Build history of the part. All positions in model axes, mm. A direction names the side the tool comes from. Give positions to 0.01 mm unless a question says otherwise; leave off trailing zeros. Order: outer loops, then holes, each group sorted by start corner. A loop starts at its lowest first (then second) coordinate and runs counter-clockwise, first axis right, second up. Notation, with made-up numbers: M -12.75,-36.5 L 13.25,-36.5 A20 ccw 13.25,-13.5 Z; hole C 58.25,-27.5 d8. An arc over 180 degrees is marked long. One line per item, written item: value.
from build123d import *

# Parameters (mm, degrees)
F1_DEPTH = 8.89


with BuildPart() as f1:
    # F0 (on Top) → F1 (new body)
    with BuildSketch(Plane.XY):
        with BuildLine():
            ThreePointArc((-31.581117, 0.265729), (-27.699647, 0.639888), (-23.961117, 1.748585))
            Line((-23.961117, 1.748585), (-23.961117, -30.38213))
            ThreePointArc((-23.961117, -30.38213), (-6.162074, -48.181174), (11.636969, -30.38213))
            Line((11.636969, -30.38213), (11.636969, -17.645674))
            ThreePointArc((11.636969, -17.645674), (8.461969, -15.95073), (5.286969, -17.645674))
            Line((5.286969, -17.645674), (5.286969, -30.38213))
            ThreePointArc((5.286969, -30.38213), (-6.162074, -41.831174), (-17.611117, -30.38213))
            Line((-17.611117, -30.38213), (-17.611117, 6.329739))
            ThreePointArc((-17.611117, 6.329739), (-12.838442, 12.752636), (-11.20179, 20.585477))
            ThreePointArc((-11.20179, 20.585477), (-31.52179, 40.905477), (-51.84179, 20.585477))
            ThreePointArc((-51.84179, 20.585477), (-48.66679, 18.093724), (-45.49179, 20.585477))
            ThreePointArc((-45.49179, 20.585477), (-21.723878, 30.34208), (-31.581117, 6.615729))
            ThreePointArc((-31.581117, 6.615729), (-33.818332, 3.440729), (-31.581117, 0.265729))
        make_face()
    extrude(amount=F1_DEPTH)


solid = f1.part
1) Saw through at B-B, the plane z = 3.25. Write the cut outline in (x, y), then the cut area to 3 significant figures.
Check values:
outline: M -51.84,20.59 A3.27 ccw -45.49,20.59 A13.91 cw long -31.58,6.62 A3.37 ccw -31.58,0.27 A20.32 ccw -23.96,1.75 L -23.96,-30.38 A17.8 ccw 11.64,-30.38 L 11.64,-17.65 A3.82 ccw 5.29,-17.65 L 5.29,-30.38 A11.45 cw -17.61,-30.38 L -17.61,6.33 A18.62 ccw -11.2,20.59 A20.32 ccw Z
area: 1,130 mm^2
2) Drill centre lines: probe 1 along X at (y, z) = (-19, 2.25); probe 2 along X at (y, z) = (-2, 4.5); probe 3 along Y at (x, z) = (-15.5, 8). Where is each one in solid material? Low to high. Write a range as from..to.
Check values:
probe 1: -23.96..-17.61, 5.29..11.64
probe 2: -23.96..-17.61
probe 3: -45.53..-37.01, 8.49..33.08
3) Saw through at A-A, the plane y = -23. Write the cut outline in (x, z), then the cut area to 3 significant figures.
Check values:
outline: M -23.96,0 L -17.61,0 L -17.61,8.89 L -23.96,8.89 Z; M 5.29,0 L 11.64,0 L 11.64,8.89 L 5.29,8.89 Z
area: 113 mm^2
4) Pin check, flat tips, straight feed: pin 1 (1 mm diameter, centred on x = 2, z = 6, fed in from -Y); pin 2 (3 mm diameter, centred on y = -31.5, z = 3.5, fed in from -X); pin 3 (4.5 mm diameter, centred on y = -8.5, z = 5.5, fed in from +X). Stop position of each tip, or through.
Check values:
pin 1: y = -46.45
pin 2: x = -23.96
pin 3: x = -17.61
5) Tool access for faces 1 (the face through (5.287, -24, 4)), 2 (the face through (11.637, -24, 4)), 3 (the face through (-5.91, -41.83, 4.38)), 4 (the face through (-48.728, 18.094, 4.383)), 5 (the face through (-12.885, 12.65, 4.383)): list every direction of +Z, -Z, +X, -X, +Y, -Y with a clear straight run to the whole face (end or side of a thin tool).
Check values:
face 1: +Z, -Z, +Y
face 2: +Z, -Z, +X, +Y, -Y
face 3: +Z, -Z
face 4: +Z, -Z, -Y
face 5: +Z, -Z, +X
6) Saw through at D-D, the plane y = -9. Write the cut outline in (x, z).
Check values:
outline: M -23.96,0 L -17.61,0 L -17.61,8.89 L -23.96,8.89 Z
7) Saw through at C-C, the plane x = -30.5. Write the cut outline in (y, z).
Check values:
outline: M 0.29,0 L 6.66,0 L 6.66,8.89 L 0.29,8.89 Z; M 34.4,0 L 40.88,0 L 40.88,8.89 L 34.4,8.89 Z
8) Mould opens along X. For faces 6 (the face through (-18, -3, 8.89)), 7 (the face through (-6.553, -48.177, 4.383)), 8 (the face through (-17.611, -12, 4)), 9 (the face through (-33.818, 3.499, 4.383)) say: released by +X, released by -X, zero draft, split by the parting line, or undercut.
Check values:
face 6: zero draft
face 7: split by the parting line
face 8: undercut
face 9: released by -X
